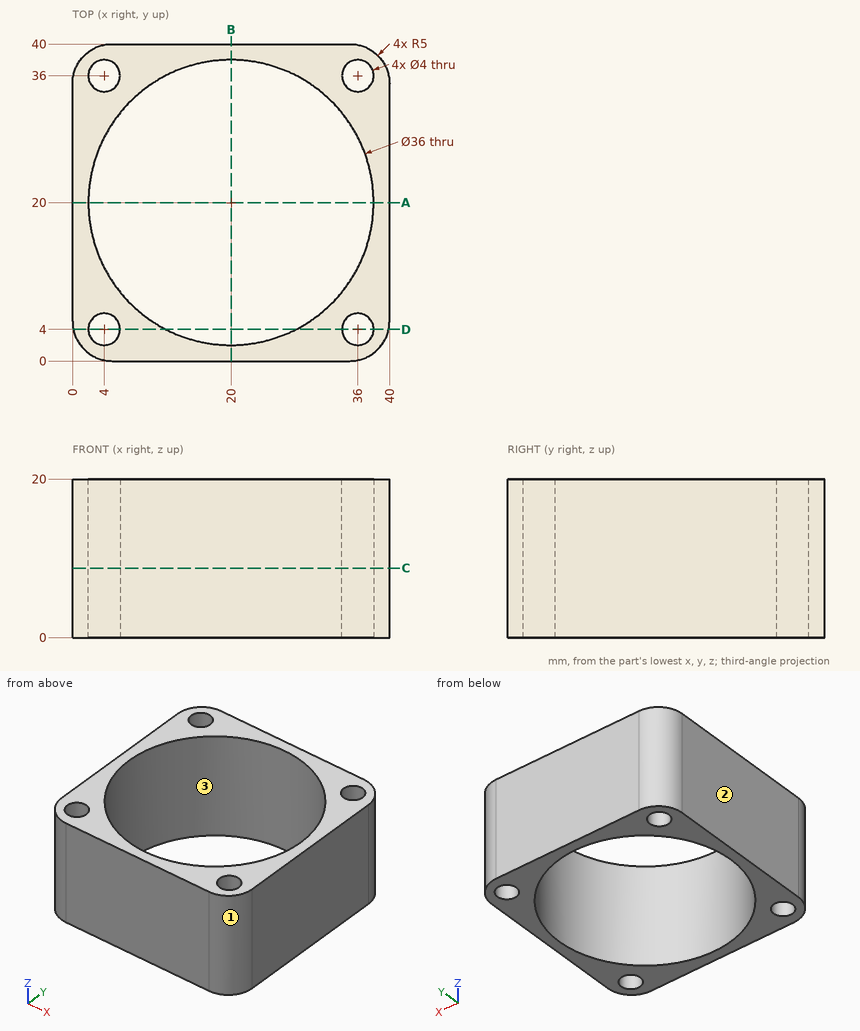
Can you work these out from the drawing? Everything is in mm from the part's minimum corner. Round coordinates to 2 decimals unless told otherwise and drop trailing zeros. Write each loop counter-clockwise with the first axis right and the second up, starting at its lowest first coordinate (ties: lowest second). Pieces come first, ordered by that corner, then holes.
1. Suppose I cut it at D-D (y = 4). List the corners of the cut face in (x, z) for me, and give its area (3 significant figures).
2. If we mould it in two halves opening along X, with no side actions, what happens to the marked faces 1, 2 and 3? For each: released by +X, released by -X, zero draft, split by the parting line, or undercut.
3. I need wall thicknesses on L1, parallel to Y at x = 36, z = 9.5; L2, parallel to X at y = 5.5, z = 12.75; L3, parallel to Y at x = 27, z = 13.5. Which ranges of each line are inside material? Lowest first, please.
4. Suppose I cut it at C-C (z = 8.75). List the corners of the cut face in (x, y) for me, and give its area (3 significant figures).
5. Suppose I cut it at A-A (y = 20). List the corners of the cut face in (x, z) for me, and give its area (3 significant figures).
Answer sheet:
1. outline: (0.1, 0) - (2, 0) - (2, 20) - (0.1, 20) - close; (6, 0) - (11.75, 0) - (11.75, 20) - (6, 20) - close; (28.25, 0) - (34, 0) - (34, 20) - (28.25, 20) - close; (38, 0) - (39.9, 0) - (39.9, 20) - (38, 20) - close
1. area: 306 mm2
2. face 1: released by +X
2. face 2: released by -X
2. face 3: undercut
3. L1: y = 0.1 to 2, 6 to 11.75, 28.25 to 34, 38 to 39.9
3. L2: x = 0 to 2.68, 5.32 to 9.33, 30.67 to 34.68, 37.32 to 40
3. L3: y = 0 to 3.42, 36.58 to 40
4. outline: (0, 5) arc R5 ccw to (5, 0) - (35, 0) arc R5 ccw to (40, 5) - (40, 35) arc R5 ccw to (35, 40) - (5, 40) arc R5 ccw to (0, 35) - close; hole circle Ø4 at (4, 4); hole circle Ø36 at (20, 20); hole circle Ø4 at (4, 36); hole circle Ø4 at (36, 4); hole circle Ø4 at (36, 36)
4. area: 510 mm2
5. outline: (0, 0) - (2, 0) - (2, 20) - (0, 20) - close; (38, 0) - (40, 0) - (40, 20) - (38, 20) - close
5. area: 80.0 mm2
